Input: part model. Units: mm. Frame: model coordinates. A direction names the side the tool comes from. Give positions to 0.01 mm unless a question says otherwise; leave off trailing zeros. Write each loop counter-clockwise with the first axis right and the second up, starting at its lowest first coordinate (ties: lowest second). Pieces come first, ordered by that corner, then holes. Notation, with made-up numbers: (1, -12.5) - (37, -12.5) arc R25 ccw to (37, 25.5) - close; hole circle Ø3 at (52, -2.75). An arc over 180 degrees is marked (long way). Answer as CSV lines item,"result".
```python
from build123d import *

# Parameters (mm, degrees)
F0_R     = 2.9
F0_R_2   = 11
F1_DEPTH = 3


with BuildPart() as f1:
    # F0 (on Top) → F1 (new body)
    with BuildSketch(Plane.XY):
        with BuildLine():
            Line((-5.24501, 29.745933), (-2.604723, 14.772116))
            ThreePointArc((-2.604723, 14.772116), (-5.130302, 14.095389), (-7.5, 12.990381))
            ThreePointArc((-7.5, 12.990381), (-9.641814, 11.490667), (-11.490667, 9.641814))
            Line((-11.490667, 9.641814), (-23.138228, 19.415279))
            ThreePointArc((-23.138228, 19.415279), (-30.5284, 17.62558), (-28.383239, 10.330654))
            Line((-28.383239, 10.330654), (-14.095389, 5.130302))
            ThreePointArc((-14.095389, 5.130302), (-14.772116, 2.604723), (-15, 0))
            ThreePointArc((-15, 0), (-14.772116, -2.604723), (-14.095389, -5.130302))
            Line((-14.095389, -5.130302), (-28.383239, -10.330654))
            ThreePointArc((-28.383239, -10.330654), (-30.5284, -17.62558), (-23.138228, -19.415279))
            Line((-23.138228, -19.415279), (-11.490667, -9.641814))
            ThreePointArc((-11.490667, -9.641814), (-9.641814, -11.490667), (-7.5, -12.990381))
            ThreePointArc((-7.5, -12.990381), (-5.130302, -14.095389), (-2.604723, -14.772116))
            Line((-2.604723, -14.772116), (-5.015594, -28.444846))
            ThreePointArc((-5.015594, -28.444846), (0, -35.25116), (5.015594, -28.444846))
            Line((5.015594, -28.444846), (2.604723, -14.772116))
            ThreePointArc((2.604723, -14.772116), (5.130302, -14.095389), (7.5, -12.990381))
            ThreePointArc((7.5, -12.990381), (9.641814, -11.490667), (11.490667, -9.641814))
            Line((11.490667, -9.641814), (22.126162, -18.566055))
            ThreePointArc((22.126162, -18.566055), (30.161985, -18.176801), (28.383239, -10.330654))
            Line((28.383239, -10.330654), (14.095389, -5.130302))
            ThreePointArc((14.095389, -5.130302), (14.772116, -2.604723), (15, 0))
            ThreePointArc((15, 0), (14.772116, 2.604723), (14.095389, 5.130302))
            Line((14.095389, 5.130302), (27.141756, 9.878791))
            ThreePointArc((27.141756, 9.878791), (30.822564, 17.032644), (23.138228, 19.415279))
            Line((23.138228, 19.415279), (11.490667, 9.641814))
            ThreePointArc((11.490667, 9.641814), (9.641814, 11.490667), (7.5, 12.990381))
            ThreePointArc((7.5, 12.990381), (5.130302, 14.095389), (2.604723, 14.772116))
            Line((2.604723, 14.772116), (5.24501, 29.745933))
            ThreePointArc((5.24501, 29.745933), (0, 35.25116), (-5.24501, 29.745933))
        make_face()
        with Locations((0, -30)):
            Circle(F0_R, mode=Mode.SUBTRACT)
        with Locations((-25.980762, -15)):
            Circle(F0_R, mode=Mode.SUBTRACT)
        with Locations((25.980762, -15)):
            Circle(F0_R, mode=Mode.SUBTRACT)
        with Locations((-25.980762, 15)):
            Circle(F0_R, mode=Mode.SUBTRACT)
        Circle(F0_R_2, mode=Mode.SUBTRACT)
        with Locations((0, 30)):
            Circle(F0_R, mode=Mode.SUBTRACT)
        with Locations((25.980762, 15)):
            Circle(F0_R, mode=Mode.SUBTRACT)
    extrude(amount=F1_DEPTH)


solid = f1.part
```
Item 1: Ray query, line 1 (Y direction, x = 2.5, z = 2.5); line 2 (Y direction, x = 1, z = 1.25); line 3 (Y direction, x = 23, z = 1.55). Return the intervals inside material, ascending. Write a range as from..to.
The answers:
line 1,"-34.62..-31.47, -28.53..-10.71, 10.71..28.53, 31.47..34.62"
line 2,"-35.16..-32.72, -27.28..-10.95, 10.95..27.28, 32.72..35.16"
line 3,"-19.32..-8.37, 8.37..19.3"
Item 2: Reachability of faces 1 (the face through (-17.4, -14.6, 1.5)), 2 (the face through (-21.139, -7.694, 1.479)), 3 (the face through (3.906, 22.154, 1.479)), 4 (the face through (-9.614, 11.514, 1.479)), 5 (the face through (20.527, 7.471, 1.479)) from +Z, -Z, +X, -X, +Y, -Y: full face, straight path, thin tool, end or side. Return the list, or none.
The answers:
face 1,"+Z, -Z, -Y"
face 2,"+Z, -Z, -X"
face 3,"+Z, -Z"
face 4,"+Z, -Z, +Y"
face 5,"+Z, -Z, +X"
Item 3: Contact query for a flat-ended pin moving along its axis: pin 1 (7.5 mm diameter, centred on x = 0, y = -30, fed in from +Z). Output: stop coordinate, or through.
The answers:
pin 1,"z = 3"
Item 4: Cut plane D-D on x = -18.5. Return the cut outline in (y, z).
The answers:
outline,"(-15.52, 0) - (-6.73, 0) - (-6.73, 3) - (-15.52, 3) - close; (6.73, 0) - (15.52, 0) - (15.52, 3) - (6.73, 3) - close"
Item 5: Cut plane B-B on y = -30. Return the cut outline in (x, z).
The answers:
outline,"(-5.25, 0) - (-2.9, 0) - (-2.9, 3) - (-5.25, 3) - close; (2.9, 0) - (5.25, 0) - (5.25, 3) - (2.9, 3) - close"
Item 6: Cut plane A-A on x = 0. Return the cut outline in (y, z), plus the area to 3 significant figures.
The answers:
outline,"(-35.25, 0) - (-32.9, 0) - (-32.9, 3) - (-35.25, 3) - close; (-27.1, 0) - (-11, 0) - (-11, 3) - (-27.1, 3) - close; (11, 0) - (27.1, 0) - (27.1, 3) - (11, 3) - close; (32.9, 0) - (35.25, 0) - (35.25, 3) - (32.9, 3) - close"
area,"111 mm²"
Item 7: Mould query, pull axis X, two halves, no side actions, for faces 6 (the face through (11, -2, 0)), 7 (the face through (-21.339, 7.767, 1.479)), 8 (the face through (-9.67, -11.467, 1.479)). Classes: +X half, -X half, draft (parallel to the pull), parting line (faces both ways), or undercut.
The answers:
face 6,"draft"
face 7,"-X half"
face 8,"undercut"
Item 8: Cut plane C-C on z = 1.6. Count the separate pieces of the cut face and the enclosed holes in it, plus the area to 3 significant figures.
The answers:
separate pieces,"1"
enclosed holes,"7"
area,"1,140 mm²"
